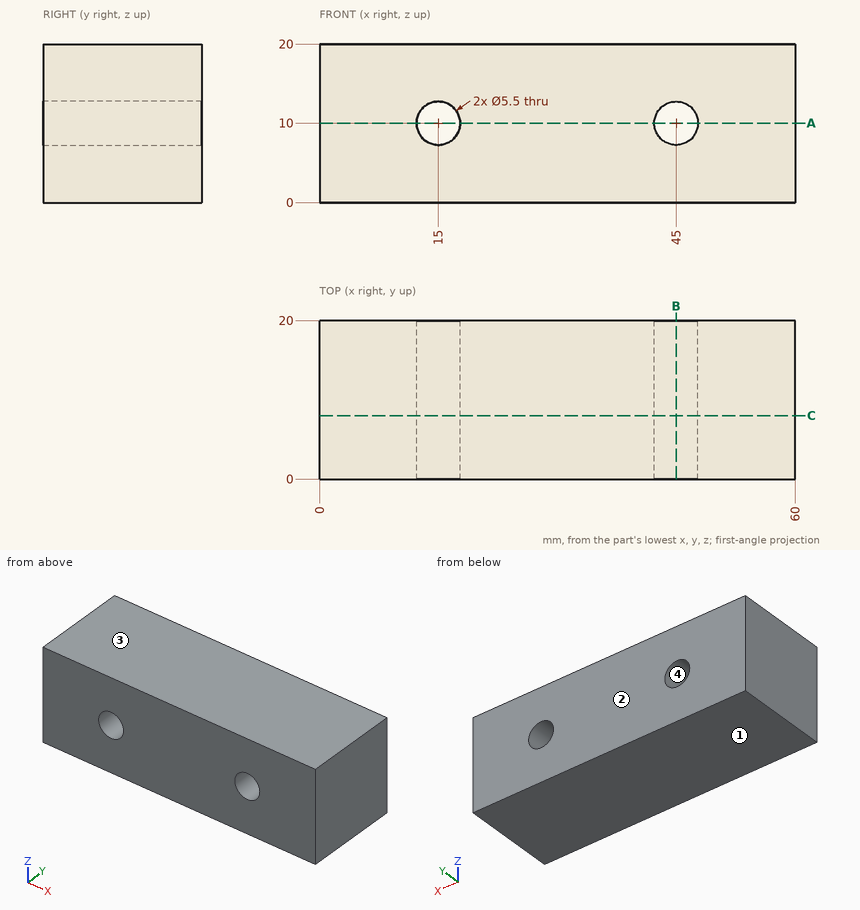
Study the drawing (mm; zero at the part's minimum x, y, z) and answer. Coordinates: 2 decimals unless noted, no trailing zeros. Write each loop counter-clockwise with the first axis right and the second up, starting at its lowest first coordinate (ties: lowest second). Pieces come first, ordered by that corner, then holes. Notation, with made-up numbers: (74.5, -12.5) - (84.5, -12.5) arc R18 ccw to (84.5, 7.5) - close; hole circle Ø7 at (21, 2.25). An arc over 180 degrees is marked (long way). One line per item, written item: value.
1) For a pull along Z with two mould halves and no side action, classify the marked faces 1, 2, 3 and 4 as pulls with the +Z half, pulls with the -Z half, needs draft (parallel to the pull), parting line crosses it, or undercut.
Geometry check:
face 1: pulls with the -Z half
face 2: needs draft
face 3: pulls with the +Z half
face 4: undercut
2) Find section C-C (y = 8). Give the vertices of the cut face in (x, z).
Geometry check:
outline: (0, 0) - (60, 0) - (60, 20) - (0, 20) - close; hole circle Ø5.5 at (15, 10); hole circle Ø5.5 at (45, 10)
3) This flat-tipped pin is pushed along its axis until it touches: pin 1 Ø3 at (y, z) = (7.5, 15.5) entering from -X. Where does it stop, or does it pass through?
Geometry check:
pin 1: stops at x = 0
4) Find section A-A (z = 10). Give the vertices of the cut face in (x, y), and give its area (3 significant figures).
Geometry check:
outline: (0, 0) - (12.25, 0) - (12.25, 20) - (0, 20) - close; (17.75, 0) - (42.25, 0) - (42.25, 20) - (17.75, 20) - close; (47.75, 0) - (60, 0) - (60, 20) - (47.75, 20) - close
area: 980 mm2
5) Consider line 1 along X through (y, z) = (15, 10); line 2 along Z through (x, y) = (15, 14.75); line 3 along X through (y, z) = (12.75, 8.5). Determine where each line is inside the solid, lowest interval first. Write a range as from..to.
Geometry check:
line 1: x = 0..12.25, 17.75..42.25, 47.75..60
line 2: z = 0..7.25, 12.75..20
line 3: x = 0..12.7, 17.3..42.7, 47.3..60
6) Find section B-B (x = 45). Give the vertices of the cut face in (y, z), and give its area (3 significant figures).
Geometry check:
outline: (0, 0) - (20, 0) - (20, 7.25) - (0, 7.25) - close; (0, 12.75) - (20, 12.75) - (20, 20) - (0, 20) - close
area: 290 mm2
